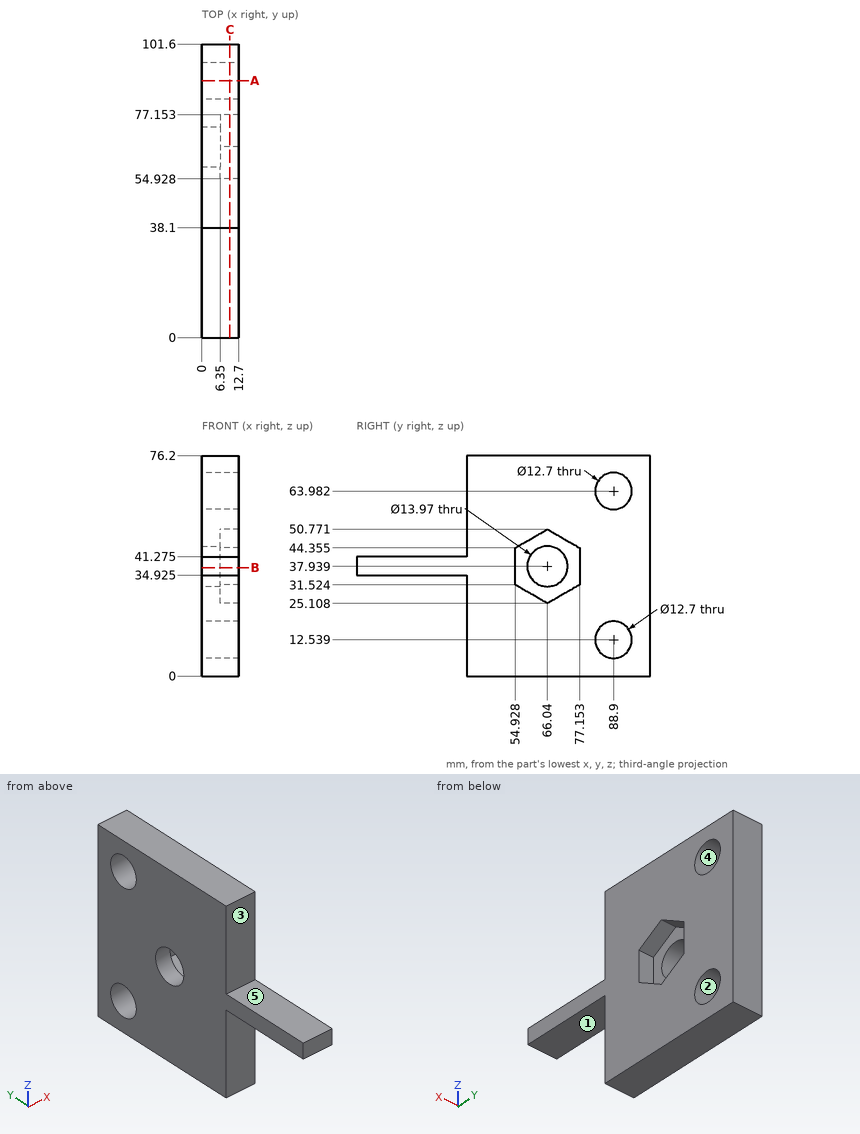
Geometry check sheet. Reference: drawing and pictorial views, mm from the part's lowest x, y, z. A direction names the side the tool comes from. Round coordinates to 2 decimals unless told otherwise and drop trailing zeros. Loops run counter-clockwise (first coordinate to the right, second up) from the corner with the lowest first, then second, coordinate; pieces in that order, holes last. Notation, with made-up numbers: M 62,9.25 L 86,9.25 A18 cw 86,32.25 Z; hole C 48.5,15 d10. An arc over 180 degrees is marked long. One line per item, written item: value.
(1) Access from +Z, -Z, +X, -X, +Y, -Y to the whole of each face (thin tool, end or side, straight path). Record for the marked faces 1 and 2.
Computed values:
face 1: -Z, +X, -X, -Y
face 2: +X, -X
(2) Release check for a two-part mould opening along Y. For the marked faces 3, 4 and 5 record: +Y half, -Y half, draft (parallel to the pull), parting line (faces both ways), or undercut.
Computed values:
face 3: -Y half
face 4: undercut
face 5: draft
(3) Depth check by flat-ended pin: pin 1 Ø3 at (x, z) = (3, 67.5) entering from -Y; pin 2 Ø6.5 at (y, z) = (62.5, 40.5) entering from +X; pin 3 Ø4 at (x, y) = (6.5, 16.5) entering from +Z (1 decimal); pin 4 Ø7.5 at (y, z) = (88.9, 63.98) entering from -X. Enter the tip coordinate at first touch or a pass-through.
Computed values:
pin 1: stops at y = 38.1
pin 2: stops at x = 6.35
pin 3: stops at z = 41.3
pin 4: passes through
(4) Sectioned sample at A-A, the plane y = 88.9. Record the cut outline in (x, z).
Computed values:
outline: M 0,0 L 12.7,0 L 12.7,6.19 L 0,6.19 Z; M 0,18.89 L 12.7,18.89 L 12.7,57.63 L 0,57.63 Z; M 0,70.33 L 12.7,70.33 L 12.7,76.2 L 0,76.2 Z
(5) Sectioned sample at C-C, the plane x = 9.75. Count the separate pieces of the cut face and the enclosed holes in it, then the cut area to 3 significant figures.
Computed values:
separate pieces: 1
enclosed holes: 3
area: 4,400 mm^2
(6) Thickness scan on line 1 (Z direction, x = 5.5, y = 88.9); line 2 (Z direction, x = 2, y = 65.5) (1 decimal); line 3 (Y direction, x = 9.25, z = 12). Record the ranges inside material, lowest first.
Computed values:
line 1: z = 0 to 6.19, 18.89 to 57.63, 70.33 to 76.2
line 2: z = 0 to 31, 44.9 to 76.2
line 3: y = 38.1 to 82.57, 95.23 to 101.6
(7) Sectioned sample at B-B, the plane z = 37.5. Record the cut outline in (x, y), then the cut area to 3 significant figures.
Computed values:
outline: M 0,0 L 12.7,0 L 12.7,54.93 L 6.35,54.93 L 6.35,59.07 L 0,59.07 Z; M 0,73.01 L 6.35,73.01 L 6.35,77.15 L 12.7,77.15 L 12.7,101.6 L 0,101.6 Z
area: 1,060 mm^2
